```python
from build123d import *

# Parameters (mm, degrees)
RESSALTO_EXTRUS_O1_DEPTH = 2
ESBO_O2_R                = 1.5
ESBO_O2_R_2              = 1
ESBO_O2_W                = 18
ESBO_O2_H                = 1.527880785
CORTE_EXTRUS_O1_DEPTH    = 3.0000001


with BuildPart() as part:
    # Esboço1 → Ressalto-extrusão1 (new body)
    with BuildSketch(Plane(origin=(0, 0, 0), x_dir=(0, 0, -1), z_dir=(1, 0, 0))):
        with BuildLine():
            Line((-13, 34), (0, 34))
            Line((0, 34), (0, -15))
            ThreePointArc((0, -15), (-12.895532653, -7.661934325), (-13.173963237, 7.172634986))
            add(Edge.make_bspline(
                [(-13, 27), (-9.354199414, 16.239964162), (-13.173963237, 7.172634986)],
                knots=[0, 0, 0, 0.912495845, 0.912495845, 0.912495845], degree=2))
            Line((-13, 27), (-13, 34))
        make_face()
    ressalto_extrus_o1 = extrude(amount=RESSALTO_EXTRUS_O1_DEPTH)

    # Espelhar1: Ressalto-extrusão1 across plane
    add(ressalto_extrus_o1.mirror(Plane(origin=(2, 34, 0), x_dir=(1, 0, 0), z_dir=(0, 0, 1))))

    # Esboço2 → Corte-extrusão1 (cut, through all)
    with BuildSketch(Plane(origin=(2, 0, 0), x_dir=(0, 0, -1), z_dir=(1, 0, 0))):
        Circle(ESBO_O2_R)
        with Locations((11, 0)):
            Circle(ESBO_O2_R_2)
        with Locations((-11, 0)):
            Circle(ESBO_O2_R_2)
        with Locations((0, 30.236059608)):
            Rectangle(ESBO_O2_W, ESBO_O2_H)
        with BuildLine():
            Line((-9.810708435, 5), (-9.219544457, 5))
            ThreePointArc((-9.219544457, 5), (-8.742813163, 5.120950927), (-8.381404052, 5.454545455))
            ThreePointArc((-8.381404052, 5.454545455), (0, 10), (8.381404052, 5.454545455))
            ThreePointArc((8.381404052, 5.454545455), (8.742813163, 5.120950927), (9.219544457, 5))
            Line((9.219544457, 5), (9.810708435, 5))
            ThreePointArc((9.810708435, 5), (10.682986811, 5.510990353), (10.663813516, 6.52173913))
            ThreePointArc((10.663813516, 6.52173913), (0, 12.5), (-10.663813516, 6.52173913))
            ThreePointArc((-10.663813516, 6.52173913), (-10.682986811, 5.510990353), (-9.810708435, 5))
        make_face()
        with BuildLine():
            Line((-9.996736389, -4.616845413), (-9.40601466, -4.639707772))
            ThreePointArc((-9.40601466, -4.639707772), (-8.934317599, -4.779005068), (-8.586080114, -5.126326976))
            ThreePointArc((-8.586080114, -5.126326976), (-0.386734657, -9.992519017), (8.164187762, -5.77460286))
            ThreePointArc((8.164187762, -5.77460286), (8.538227759, -5.455234837), (9.019280003, -5.352811245))
            Line((9.019280003, -5.352811245), (9.610001733, -5.375673604))
            ThreePointArc((9.610001733, -5.375673604), (10.461865791, -5.920015714), (10.403617681, -6.929266854))
            ThreePointArc((10.403617681, -6.929266854), (-0.483418321, -12.490648771), (-10.90805419, -6.104453603))
            ThreePointArc((-10.90805419, -6.104453603), (-10.888123983, -5.093719467), (-9.996736389, -4.616845413))
        make_face()
    extrude(amount=-CORTE_EXTRUS_O1_DEPTH, mode=Mode.SUBTRACT)


solid = part.part
```
Input: part model. Units: mm. Frame: model coordinates. A direction names the side the tool comes from. Coordinates: 2 decimals unless noted, no trailing zeros. Loops run counter-clockwise (first coordinate to the right, second up) from the corner with the lowest first, then second, coordinate; pieces in that order, holes last. Notation, with made-up numbers: M -13,-24.5 L 9,-24.5 A22 ccw 9,-5.5 Z; hole C 45,-13 d5. An arc over 180 degrees is marked long. Use a Markdown table: item, result. Add a question column.
1) Section D-D, the plane x = 1.6. Give the number of separate pieces and of enclosed holes in the cut face, plus the area to 3 significant figures.
2) Line query: L1, parallel to Y at x = 0.5, z = 0; L2, parallel to Y at x = 0.55, z = 3; L3, parallel to Y at x = 1.5, z = 2.5. Output: solid intervals per line, ascending. Write a range as from..to.
3) Set-up query: faces 1 (the flat face through (1, 30, -13)), 2 (the cylindrical face through (1.014, -5.907, -10.455)), 3 (the flat face through (1, 34, 0)). Return all of +Z, -Z, +X, -X, +Y, -Y with unobstructed straight access to the full face (end or side cutting, diameter ignored); none if empty.
4) Pin query (flat end, axial travel): P1, Ø0.5, axis at x = 1.5, y = 30, coming from the -Z side; P2, Ø0.6, axis at x = 1.5, y = 30, coming from the +Z side; P3, Ø0.6, axis at x = 1, z = 1, coming from the -Y side. Return the tip coordinate at first contact, or that it passes through.
5) Draft query along Z for faces 4 (the flat face through (0, 9.8, 0.2)), 5 (the flat face through (1, 30, 13)), 6 (the flat face through (1, 29.472, 0)). Return one class per face: +Z half, -Z half, draft (parallel to the pull), parting line (faces both ways), or undercut.
6) Section B-B, the plane z = 6. Return the cut outline in (x, y).
7) Section A-A, the plane y = 0. Return the cut outline in (x, z).
8) Section C-C, the plane y = 30. Return the cut outline in (x, z).
Answer below:
| question | item | result |
|---|---|---|
| 1 | separate pieces | 1 |
| 1 | enclosed holes | 6 |
| 1 | area | 1,050 mm2 |
| 2 | L1 | -15..-12.5, -10..-1.5, 1.5..10, 12.5..29.47, 31..34 |
| 2 | L2 | -14.7..-12.13, -9.54..9.54, 12.13..29.47, 31..34 |
| 2 | L3 | -14.79..-12.25, -9.68..9.68, 12.25..29.47, 31..34 |
| 3 | face 1 | -Z, +X, -X, +Y |
| 3 | face 2 | +X, -X |
| 3 | face 3 | +Z, -Z, +X, -X, +Y |
| 4 | P1 | z = -13 |
| 4 | P2 | z = 13 |
| 4 | P3 | y = -14.98 |
| 5 | face 4 | draft |
| 5 | face 5 | +Z half |
| 5 | face 6 | undercut |
| 6 | outline | M 0,-13.75 L 2,-13.75 L 2,-10.97 L 0,-10.97 Z; M 0,-8 L 2,-8 L 2,8 L 0,8 Z; M 0,10.97 L 2,10.97 L 2,29.47 L 0,29.47 Z; M 0,31 L 2,31 L 2,34 L 0,34 Z |
| 7 | outline | M 0,-15 L 2,-15 L 2,-12 L 0,-12 Z; M 0,-10 L 2,-10 L 2,-1.5 L 0,-1.5 Z; M 0,1.5 L 2,1.5 L 2,10 L 0,10 Z; M 0,12 L 2,12 L 2,15 L 0,15 Z |
| 8 | outline | M 0,-13 L 2,-13 L 2,-9 L 0,-9 Z; M 0,9 L 2,9 L 2,13 L 0,13 Z |
